```python
from build123d import *

# Parameters (mm, degrees)
SKETCH1_W                   = 19.05
SKETCH1_H                   = 3.175
EXTRUDE1_DEPTH              = 25.4
CUT_EXTRUDE1_DEPTH          = 28.312382723
CHAMFER1_SIZE               = 6.35
F_1_4_0_25_DIAMETER_HOLE1_D = 6.35
FILLET1_R                   = 1.5875


with BuildPart() as part:
    # Sketch1 → Extrude1 (new, symmetric)
    with BuildSketch(Plane.XY):
        Rectangle(SKETCH1_W, SKETCH1_H)
    extrude(amount=EXTRUDE1_DEPTH, both=True)

    # Sketch2 → Cut-Extrude1 (cut, through all)
    with BuildSketch(Plane(origin=(0, 1.5875, 0), x_dir=(-1, 0, 0), z_dir=(0, 1, 0))):
        with BuildLine():
            Line((3.571875, -17.4625), (3.571875, 11.1125))
            ThreePointArc((3.571875, 11.1125), (0, 14.684375), (-3.571875, 11.1125))
            Line((-3.571875, 11.1125), (-3.571875, -17.4625))
            ThreePointArc((-3.571875, -17.4625), (0, -21.034375), (3.571875, -17.4625))
        make_face()
    extrude(amount=-CUT_EXTRUDE1_DEPTH, mode=Mode.SUBTRACT)

    # Chamfer1
    chamfer1_edges = [part.edges().sort_by_distance(p)[0] for p in [
        (9.525, 0, 25.4),
        (-9.525, 0, 25.4),
    ]]
    chamfer(chamfer1_edges, length=CHAMFER1_SIZE)

    # 1/4 (0.25) Diameter Hole1 (through all)
    with Locations(Plane(origin=(0, 1.5875, 0), x_dir=(-1, 0, 0), z_dir=(0, 1, 0))):
        with Locations((0, 20.6375)):
            Hole(F_1_4_0_25_DIAMETER_HOLE1_D / 2)

    # Fillet1
    fillet1_edges = [part.edges().sort_by_distance(p)[0] for p in [
        (3.175, 0, 25.4),
        (-3.175, 0, 25.4),
        (-9.525, 0, 19.05),
        (9.525, 0, 19.05),
        (9.525, 0, -25.4),
        (-9.525, 0, -25.4),
    ]]
    fillet(fillet1_edges, radius=FILLET1_R)


solid = part.part
```
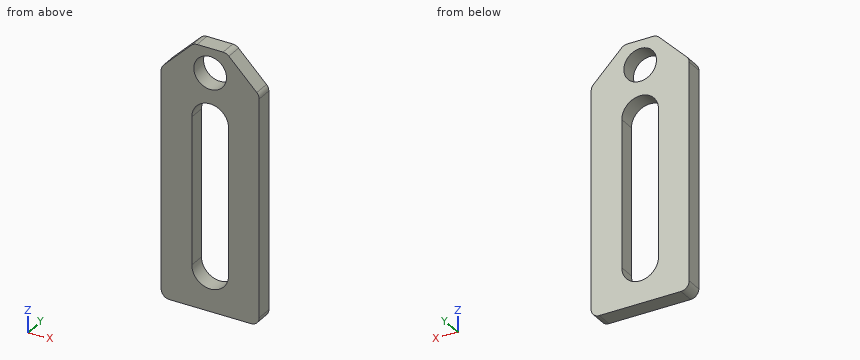
Verification items for the finished model (mm, model axes). Coordinates: 2 decimals unless noted, no trailing zeros. Order: outer loops, then holes, each group sorted by start corner. A loop starts at its lowest first (then second) coordinate and runs counter-clockwise, first axis right, second up. Notation, with made-up numbers: (59, 79) - (111, 79) arc R12 ccw to (111, 90) - close; hole circle Ø8 at (12.25, 72.25). An arc over 180 degrees is marked (long way). Return JSON: item names as keys, results as strings.
(1) Section check A-A, the plane z = -16. Record the cut outline in (x, y) (1 decimal), and give its area (3 significant figures).
Filled sheet:
{"outline": "(-9.5, -1.6) - (-3.6, -1.6) - (-3.6, 1.6) - (-9.5, 1.6) - close; (3.6, -1.6) - (9.5, -1.6) - (9.5, 1.6) - (3.6, 1.6) - close", "area": "37.8 mm^2"}
(2) Section check B-B, the plane x = 0. Record the cut outline in (y, z), and give its area (3 significant figures).
Filled sheet:
{"outline": "(-1.59, -25.4) - (1.59, -25.4) - (1.59, -21.03) - (-1.59, -21.03) - close; (-1.59, 14.68) - (1.59, 14.68) - (1.59, 17.46) - (-1.59, 17.46) - close; (-1.59, 23.81) - (1.59, 23.81) - (1.59, 25.4) - (-1.59, 25.4) - close", "area": "27.7 mm^2"}
(3) Section check C-C, the plane y = -0.7. Give the number of separate pieces and of enclosed holes in the cut face, and give its area (3 significant figures).
Filled sheet:
{"separate pieces": "1", "enclosed holes": "2", "area": "650 mm^2"}
(4) Go/stop test with a flat-tipped pin: pin 1 (7.5 mm diameter, centred on x = 0, z = 20.64, fed in from -Y). Record where the tip stops, or that it passes through.
Filled sheet:
{"pin 1": "stops at y = -1.59"}
(5) Thickness scan on line 1 along Z through (x, y) = (0, 0.65); line 2 along Z through (x, y) = (-2, 0.75); line 3 along X through (y, z) = (0, -5) (3 decimals). Record the ranges inside material, lowest first.
Filled sheet:
{"line 1": "z = -25.4 to -21.03, 14.68 to 17.46, 23.81 to 25.4", "line 2": "z = -25.4 to -20.42, 14.07 to 18.17, 23.1 to 25.4", "line 3": "x = -9.525 to -3.572, 3.572 to 9.525"}
(6) Section check D-D, the plane z = 20. Record the cut outline in (x, y) (1 decimal).
Filled sheet:
{"outline": "(-8.6, -1.6) - (-3.1, -1.6) - (-3.1, 1.6) - (-8.6, 1.6) - close; (3.1, -1.6) - (8.6, -1.6) - (8.6, 1.6) - (3.1, 1.6) - close"}
